```python
from build123d import *

# Parameters (mm, degrees)
SKETCH1_W           = 431.8
SKETCH1_H           = 171.45
BOSS_EXTRUDE1_DEPTH = 85.725
CUT_EXTRUDE1_DEPTH  = 73.025
CHAMFER1_SIZE       = 0.635


with BuildPart() as part:
    # Sketch1 → Boss-Extrude1 (new body)
    with BuildSketch(Plane(origin=(0, 0, 0), x_dir=(1, 0, 0), z_dir=(0, 1, 0))):
        Rectangle(SKETCH1_W, SKETCH1_H)
    extrude(amount=BOSS_EXTRUDE1_DEPTH)

    # Sketch2 → Cut-Extrude1 (cut)
    with BuildSketch(Plane.XZ):
        with BuildLine():
            Line((178.806416914, 72.140394915), (-178.806416914, 72.140394915))
            ThreePointArc((-178.806416914, 72.140394915), (-195.429774677, 65.254774677), (-202.315394915, 48.631416914))
            Line((-202.315394915, 48.631416914), (-202.315394915, -48.631416914))
            ThreePointArc((-202.315394915, -48.631416914), (-195.429774677, -65.254774677), (-178.806416914, -72.140394915))
            Line((-178.806416914, -72.140394915), (178.806416914, -72.140394915))
            ThreePointArc((178.806416914, -72.140394915), (195.429774677, -65.254774677), (202.315394915, -48.631416914))
            Line((202.315394915, -48.631416914), (202.315394915, 48.631416914))
            ThreePointArc((202.315394915, 48.631416914), (195.429774677, 65.254774677), (178.806416914, 72.140394915))
        make_face()
    extrude(amount=-CUT_EXTRUDE1_DEPTH, mode=Mode.SUBTRACT)

    # Chamfer1
    chamfer1_edges = [part.edges().sort_by_distance(p)[0] for p in [
        (195.429774677, 0, 65.254774677),
        (195.429774677, 0, -65.254774677),
        (-195.429774677, 0, -65.254774677),
        (0, 0, 72.140394915),
        (-195.429774677, 0, 65.254774677),
        (-202.315394915, 0, 0),
        (0, 0, -72.140394915),
        (202.315394915, 0, 0),
    ]]
    chamfer(chamfer1_edges, length=CHAMFER1_SIZE)


solid = part.part
```
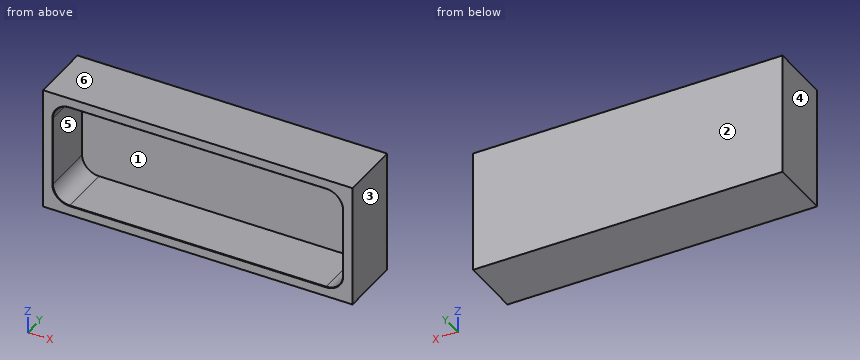
Input: part model. Units: mm. Frame: model coordinates. Face numbers are marked on the shaded views. A direction names the side the tool comes from. Round coordinates to 2 decimals unless told otherwise and drop trailing zeros. Loops run counter-clockwise (first coordinate to the right, second up) from the corner with the lowest first, then second, coordinate; pieces in that order, holes last.
1) Set-up query: the marked faces 5 and 6. Return all of +Z, -Z, +X, -X, +Y, -Y with unobstructed straight access to the full face (end or side cutting, diameter ignored); none if empty.
Ans:
face 5: -Y
face 6: +Z, +X, -X, +Y, -Y
2) Section query C-C on x = 46. Return the cut outline in (y, z) (3 decimals).
Ans:
outline: (0, -85.725) - (85.725, -85.725) - (85.725, 85.725) - (0, 85.725) - (0, 72.775) - (0.635, 72.14) - (73.025, 72.14) - (73.025, -72.14) - (0.635, -72.14) - (0, -72.775) - close
3) Pin query (flat end, axial travel): pin 1 (5 mm diameter, centred on x = -116, z = 55.5, fed in from -Y) (3 decimals). Return the tip coordinate at first contact, or that it passes through.
Ans:
pin 1: stops at y = 73.025
4) Pull-direction query (X, two-part tool) for the marked faces 1, 2, 3 and 4; classes: released by +X, released by -X, zero draft, split by the parting line, or undercut.
Ans:
face 1: undercut
face 2: zero draft
face 3: released by +X
face 4: released by -X
5) Material intervals for line 1 (Z direction, x = 161.5, y = 59) (3 decimals); line 2 (X direction, y = 20.5, z = -27); line 3 (Y direction, x = 103.5, z = -31) (3 decimals), sorted ascending.
Ans:
line 1: z = -85.725 to -72.14, 72.14 to 85.725
line 2: x = -215.9 to -202.32, 202.32 to 215.9
line 3: y = 73.025 to 85.725
6) Section query B-B on z = 6. Return the cut outline in (x, y) (3 decimals).
Ans:
outline: (-215.9, 0) - (-202.95, 0) - (-202.315, 0.635) - (-202.315, 73.025) - (202.315, 73.025) - (202.315, 0.635) - (202.95, 0) - (215.9, 0) - (215.9, 85.725) - (-215.9, 85.725) - close
7) Section query A-A on y = 63. Return the cut outline in (x, z) (3 decimals), plus the area to 3 significant figures.
Ans:
outline: (-215.9, -85.725) - (215.9, -85.725) - (215.9, 85.725) - (-215.9, 85.725) - close; hole (-202.315, -48.631) arc R23.509 ccw to (-178.806, -72.14) - (178.806, -72.14) arc R23.509 ccw to (202.315, -48.631) - (202.315, 48.631) arc R23.509 ccw to (178.806, 72.14) - (-178.806, 72.14) arc R23.509 ccw to (-202.315, 48.631) - close
area: 16,100 mm2
